Read the model definition and answer for the solid it produces. Units are mm, in the model's axes. A direction names the side the tool comes from. Coordinates: 2 decimals unless noted, no trailing zeros. Write each loop counter-clockwise with the first axis right and the second up, starting at its lowest first coordinate (ties: lowest second). Pieces come first, ordered by that corner, then holes. Notation, with made-up numbers: (-7.75, -30) -> (49.25, -30) arc R10 cw to (49.25, -11) -> close; hole circle Ø1 at (2, 41.25). An arc over 180 degrees is marked (long way). Answer in a Markdown table with one row per item. Add a question column.
Item 1: Section A-A on y = 1 is taken. Write down the section's boundary in (x, z).
Item 2: Which of the six approach directions +Z, -Z, +X, -X, +Y, -Y give full straight-line access (tool end or side, diameter ignored) to faces 1 (the face through (1.94, 0.74, 1.14)), 2 (the face through (1, 1.5, -1))?
Item 3: Section B-B on y = 3.25 is taken. Write down the section's boundary in (x, z).
Item 4: Straight lines are drawn through the part: line 1 (Z direction, x = -0.05, y = 3.25); line 2 (Y direction, x = 0.9, z = 0.7); line 3 (Z direction, x = -0.8, y = 7.75). For each, find the intervals that lie inside material, in ascending order. Write a range as from..to.
Item 5: Given pin 1 Ø2 at (x, y) = (0.5, 7) entering from +Z; pin 2 Ø1 at (x, y) = (2, 9) entering from -Z; pin 3 Ø1.5 at (y, z) = (4.5, -1.5) entering from +X, each flat-ended and moving along its own axis, determine where each tip first touches the part or whether it passes through.
```python
from build123d import *

# Parameters (mm, degrees)
BOSS_EXTRUDE2_DEPTH = 1.5
SKETCH2_OUTSIDE_W   = 13.8
SKETCH2_OUTSIDE_H   = 13.104
SKETCH2_OUTSIDE_R   = 2.25
CUT_EXTRUDE1_DEPTH  = 1.5
CUT_EXTRUDE1_TAPER  = 60
SKETCH3_R           = 1
BOSS_EXTRUDE3_DEPTH = 9
FILLET1_R           = 0.1
FILLET2_R           = 0.15


with BuildPart() as part:
    # Sketch1 → Boss-Extrude2 (new body)
    with BuildSketch(Plane(origin=(0, 0, 0), x_dir=(1, 0, 0), z_dir=(0, 1, 0))):
        Polygon((2.598076211, 0), (1.299038106, 2.25), (-1.299038106, 2.25), (-2.598076211, 0), (-1.299038106, -2.25), (1.299038106, -2.25), align=None)
    extrude(amount=BOSS_EXTRUDE2_DEPTH)

    # Sketch2 outside → Cut-Extrude1 (cut)
    with BuildSketch(Plane(origin=(0, 0, 0), x_dir=(1, 0, 0), z_dir=(0, 1, 0))):
        Rectangle(SKETCH2_OUTSIDE_W, SKETCH2_OUTSIDE_H)
        Circle(SKETCH2_OUTSIDE_R, mode=Mode.SUBTRACT)
    extrude(amount=CUT_EXTRUDE1_DEPTH, taper=CUT_EXTRUDE1_TAPER, mode=Mode.SUBTRACT)

    # Sketch3 → Boss-Extrude3 (add)
    with BuildSketch(Plane(origin=(0, 1.5, 0), x_dir=(1, 0, 0), z_dir=(0, 1, 0))):
        Circle(SKETCH3_R)
    extrude(amount=BOSS_EXTRUDE3_DEPTH)

    # Fillet1
    fillet1_edges = [part.edges().sort_by_distance(p)[0] for p in [
        (-1, 10.5, 0),
    ]]
    fillet(fillet1_edges, radius=FILLET1_R)

    # Fillet2
    fillet2_edges = [part.edges().sort_by_distance(p)[0] for p in [
        (-1, 1.5, 0),
    ]]
    fillet(fillet2_edges, radius=FILLET2_R)


solid = part.part
```
Results below:
| question | item | result |
|---|---|---|
| 1 | outline | (-2.6, 0) -> (-1.3, -2.25) -> (1.3, -2.25) -> (2.6, 0) -> (1.3, 2.25) -> (-1.3, 2.25) -> close |
| 2 | face 1 | +Z, +X, +Y, -Y |
| 2 | face 2 | +Y |
| 3 | outline | circle Ø2 at (0, 0) |
| 4 | line 1 | z = -1..1 |
| 4 | line 2 | y = 0..1.5 |
| 4 | line 3 | z = -0.6..0.6 |
| 5 | pin 1 | stops at z = 1 |
| 5 | pin 2 | passes through |
| 5 | pin 3 | stops at x = 0.66 |
